For this review, use the dimensioned drawing (mm, ordinates from the lowest corner) and the shaded views. A direction names the side the tool comes from. Round coordinates to 2 decimals unless told otherwise and drop trailing zeros. Order: outer loops, then holes, each group sorted by start corner. A loop starts at its lowest first (then second) coordinate and runs counter-clockwise, first axis right, second up. Notation, with made-up numbers: (6, 82) - (18, 82) arc R29 cw to (18, 102) - close; hole circle Ø3 at (82, 73). An arc over 180 degrees is marked (long way). Use CSV: the item, a comma, the result in double quotes. Start each with the question number.
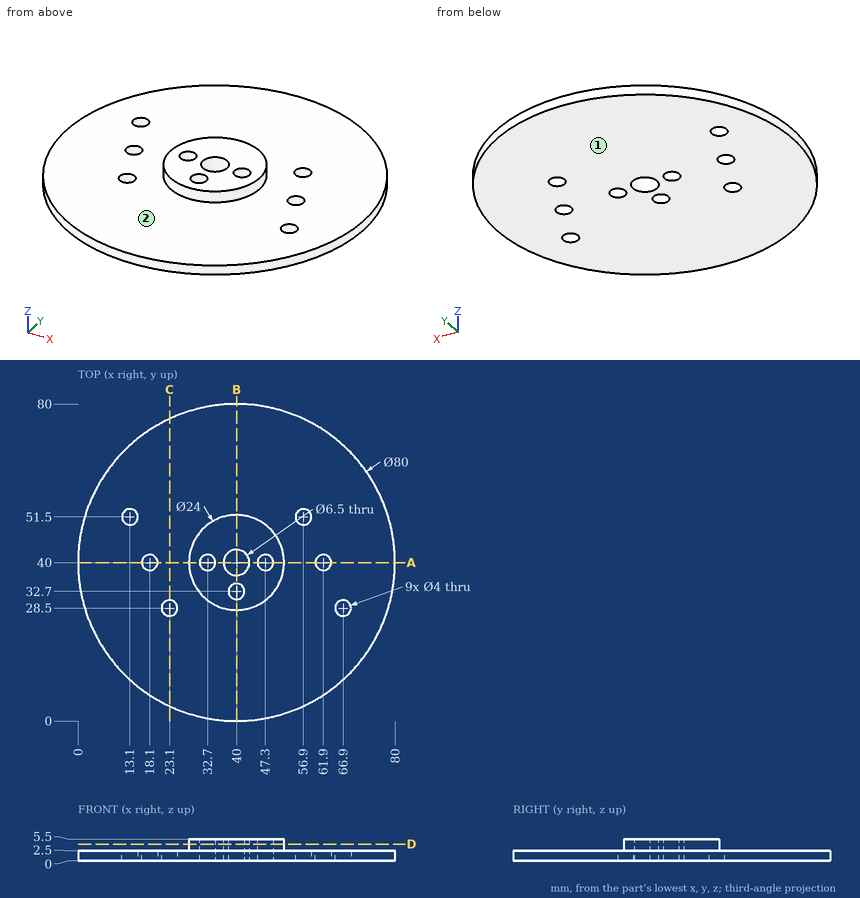
Q1. Take a section at D-D (z = 4.2). State the section outline as (x, y) points.
Q2. Take a section at B-B (x = 40). State the section outline as (y, z) points.
Q3. Clearance check with flat-ended pins moving along their axes: pin 1 (2.5 mm diameter, centred on x = 40, y = 32.7, fed in from +Z); pin 2 (1 mm diameter, centred on x = 40.5, z = 1.5, fed in from -Y); pin 3 (1 mm diameter, centred on x = 58.5, y = 49.5, fed in from +Z); pin 4 (1 mm diameter, centred on y = 36.5, z = 1.5, fed in from +X). State where each tip first meets the part, or that it passes through.
Q4. For L1, parallel to X at y = 39, z = 3.1; L2, parallel to Z at x = 24.5, y = 60; L3, parallel to Y at x = 56.9, z = 0.7, list the stretches that pass through material, from the lowest coordinate up. Write a range as [from, to].
Q5. Take a section at C-C (x = 23.1). State the section outline as (y, z) points, plus the area to 3 significant figures.
Q6. Take a section at A-A (y = 40). State the section outline as (x, z) points.
Q7. Tool access review of the marked faces 1 and 2: name each direction out of +Z, -Z, +X, -X, +Y, -Y from which nothing blocks a thin tool from reaching the whole face with its end or side.
Findings below:
1,outline,"circle Ø24 at (40, 40); hole circle Ø4 at (32.7, 40); hole circle Ø6.5 at (40, 40); hole circle Ø4 at (40, 32.7); hole circle Ø4 at (47.3, 40)"
2,outline,"(0, 0) - (30.7, 0) - (30.7, 5.5) - (28, 5.5) - (28, 2.5) - (0, 2.5) - close; (34.7, 0) - (36.75, 0) - (36.75, 5.5) - (34.7, 5.5) - close; (43.25, 0) - (80, 0) - (80, 2.5) - (52, 2.5) - (52, 5.5) - (43.25, 5.5) - close"
3,pin 1,"passes through"
3,pin 2,"stops at y = 0"
3,pin 3,"stops at z = 2.5"
3,pin 4,"stops at x = 79.89"
4,L1,"x = [28.04, 30.97], [34.43, 36.91], [43.09, 45.57], [49.03, 51.96]"
4,L2,"z = [0, 2.5]"
4,L3,"y = [3.75, 49.5], [53.5, 76.25]"
5,outline,"(3.75, 0) - (26.5, 0) - (26.5, 2.5) - (3.75, 2.5) - close; (30.5, 0) - (76.25, 0) - (76.25, 2.5) - (30.5, 2.5) - close"
5,area,"171 mm^2"
6,outline,"(0, 0) - (16.1, 0) - (16.1, 2.5) - (0, 2.5) - close; (20.1, 0) - (30.7, 0) - (30.7, 5.5) - (28, 5.5) - (28, 2.5) - (20.1, 2.5) - close; (34.7, 0) - (36.75, 0) - (36.75, 5.5) - (34.7, 5.5) - close; (43.25, 0) - (45.3, 0) - (45.3, 5.5) - (43.25, 5.5) - close; (49.3, 0) - (59.9, 0) - (59.9, 2.5) - (52, 2.5) - (52, 5.5) - (49.3, 5.5) - close; (63.9, 0) - (80, 0) - (80, 2.5) - (63.9, 2.5) - close"
7,face 1,"-Z, +X, -X, +Y, -Y"
7,face 2,"+Z"
